from build123d import *

# Parameters (mm, degrees)
SKETCH_1_R          = 12.5
EXTRUDE_1_DEPTH     = 4
SKETCH_2_R          = 12.5
SKETCH_2_R_2        = 10
EXTRUDE_2_DEPTH     = 2.5
SKETCH_3_R          = 1.5
CUT_EXTRUDE_1_DEPTH = 52.947088465
EXTRUDE_3_DEPTH     = 25
SKETCH_5_W          = 7
SKETCH_5_H          = 5
CUT_EXTRUDE_2_DEPTH = 57.621550668
SKETCH_6_W          = 7
SKETCH_6_H          = 5
CUT_EXTRUDE_3_DEPTH = 52.780787943
EXTRUDE_6_DEPTH     = 2


with BuildPart() as part:
    # 草图1 → 凸台-拉伸1 (new body)
    with BuildSketch(Plane(origin=(0, 0, 0), x_dir=(1, 0, 0), z_dir=(0, 1, 0))):
        Circle(SKETCH_1_R)
        with BuildLine():
            Line((50, 12.5), (0, 12.5))
            ThreePointArc((0, 12.5), (8.838834765, 8.838834765), (12.5, 0))
            ThreePointArc((12.5, 0), (8.838834765, -8.838834765), (0, -12.5))
            Line((0, -12.5), (50, -12.5))
            Line((50, -12.5), (50, 12.5))
        make_face()
    extrude(amount=EXTRUDE_1_DEPTH)

    # 草图2 → 凸台-拉伸2 (add)
    with BuildSketch(Plane(origin=(0, 4, 0), x_dir=(1, 0, 0), z_dir=(0, 1, 0))):
        with Locations(Location((0, 0, 0), (0, 0, 270))):
            Circle(SKETCH_2_R)
        with Locations(Location((0, 0, 0), (0, 0, 270))):
            Circle(SKETCH_2_R_2, mode=Mode.SUBTRACT)
    extrude(amount=EXTRUDE_2_DEPTH)

    # 草图3 → 切除-拉伸1 (cut, through all)
    with BuildSketch(Plane.XZ):
        with Locations(Location((0, 0, 0), (0, 0, 270))):
            Circle(SKETCH_3_R)
        with Locations(Location((0, 7, 0), (0, 0, 270))):
            Circle(SKETCH_3_R)
        with Locations(Location((7, 0, 0), (0, 0, 270))):
            Circle(SKETCH_3_R)
        with Locations(Location((0, -7, 0), (0, 0, 270))):
            Circle(SKETCH_3_R)
        with Locations(Location((-7, 0, 0), (0, 0, 270))):
            Circle(SKETCH_3_R)
        with Locations(Location((40, 0, 0), (0, 0, 270))):
            Circle(SKETCH_3_R)
    extrude(amount=-CUT_EXTRUDE_1_DEPTH, mode=Mode.SUBTRACT)

    # 草图4 → 凸台-拉伸3 (add)
    with BuildSketch(Plane.XY.offset(12.5)):
        Polygon((50, 4), (47, 9), (33, 9), (30, 4), align=None)
    extrude(amount=-EXTRUDE_3_DEPTH)

    # 草图5 → 切除-拉伸2 (cut, through all)
    with BuildSketch(Plane.XY.offset(12.5)):
        with Locations((40, 6.5)):
            Rectangle(SKETCH_5_W, SKETCH_5_H)
    extrude(amount=-CUT_EXTRUDE_2_DEPTH, mode=Mode.SUBTRACT)

    # 草图6 → 切除-拉伸3 (cut, through all)
    with BuildSketch(Plane(origin=(0, 4, 0), x_dir=(1, 0, 0), z_dir=(0, 1, 0))):
        with Locations((40, -10)):
            Rectangle(SKETCH_6_W, SKETCH_6_H)
        with Locations((40, 10)):
            Rectangle(SKETCH_6_W, SKETCH_6_H)
    extrude(amount=-CUT_EXTRUDE_3_DEPTH, mode=Mode.SUBTRACT)

    # 草图7 → 凸台-拉伸6 (add, symmetric)
    with BuildSketch(Plane.XY):
        Polygon((30, 4), (33, 9), (12.5, 6.5), (10.351420614, 6.5), (10.351420614, 4), align=None)
    extrude(amount=EXTRUDE_6_DEPTH, both=True)


solid = part.part
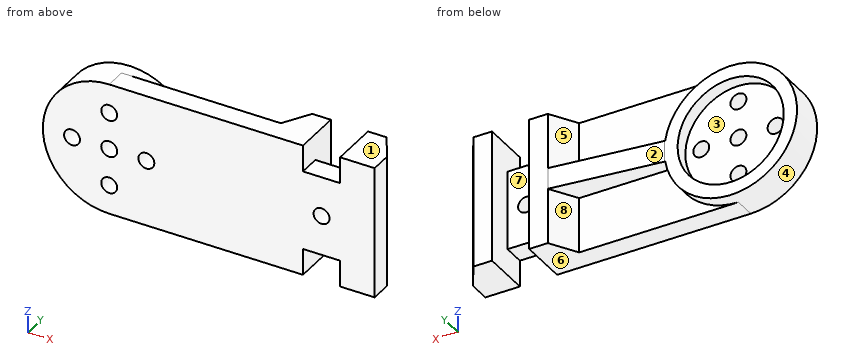
Verification items for the finished model (mm, model axes). Face numbers are marked on the shaded views. A direction names the side the tool comes from. Round coordinates to 2 decimals unless told otherwise and drop trailing zeros. Order: outer loops, then holes, each group sorted by start corner. A loop starts at its lowest first (then second) coordinate and runs counter-clockwise, first axis right, second up.
1. Section check D-D on z = -6.5. Record the cut outline in (x, y).
Final values:
outline: (-10.68, 0) - (-1.41, 0) - (-1.41, 4) - (-7.6, 4) - (-7.6, 6.5) - (-10.68, 6.5) - close; (1.41, 0) - (50, 0) - (50, 4) - (47, 9) - (43.5, 9) - (43.5, 4) - (36.5, 4) - (36.5, 9) - (33, 9) - (30, 4) - (10.68, 4) - (10.68, 6.5) - (7.6, 6.5) - (7.6, 4) - (1.41, 4) - close
2. Release check for a two-part mould opening along X. For the marked faces 1, 2 and 3 record: +X half, -X half, draft (parallel to the pull), parting line (faces both ways), or undercut.
Final values:
face 1: draft
face 2: -X half
face 3: undercut
3. Go/stop test with flat-tipped pins: P1, Ø4, axis at x = 26.5, y = 7, coming from the -Z side; P2, Ø1.5, axis at x = 26.5, y = 6, coming from the +Z side; P3, Ø2, axis at y = 6, z = 8, coming from the +X side. Record where each tip stops, or that it passes through.
Final values:
P1: stops at z = -2
P2: stops at z = 2
P3: stops at x = 49.4
4. Section check B-B on z = 0. State how many separate pieces and enclosed holes the cut face has, then the cut area to 3 significant figures.
Final values:
separate pieces: 5
enclosed holes: 0
area: 334 mm2
5. Thickness scan on L1, parallel to X at y = 2.45, z = 0; L2, parallel to Y at x = 24, z = -6.5; L3, parallel to X at y = 2.25, z = -7. Record the ranges inside material, lowest first.
Final values:
L1: x = -12.5 to -8.5, -5.5 to -1.5, 1.5 to 5.5, 8.5 to 38.5, 41.5 to 50
L2: y = 0 to 4
L3: x = -10.36 to -1.5, 1.5 to 50
6. Section check C-C on x = 40. Record the cut outline in (y, z), then the cut area to 3 significant figures.
Final values:
outline: (0, -7.5) - (4, -7.5) - (4, -1.5) - (0, -1.5) - close; (0, 1.5) - (4, 1.5) - (4, 7.5) - (0, 7.5) - close
area: 48.0 mm2
7. Section check A-A on y = 5. Record the cut outline in (x, z).
Final values:
outline: (12.34, -2) - (30.6, -2) - (30.6, -12.5) - (36.5, -12.5) - (36.5, 12.5) - (30.6, 12.5) - (30.6, 2) - (12.34, 2) arc R12.5 ccw (long way) to start; (43.5, -12.5) - (49.4, -12.5) - (49.4, 12.5) - (43.5, 12.5) - close; hole circle Ø20 at (0, 0)
8. Access from +Z, -Z, +X, -X, +Y, -Y to the whole of each face (thin tool, end or side, straight path). Record for the marked faces 4, 5, 6, 7 and 8.
Final values:
face 4: +Y
face 5: +Z, +Y
face 6: -Z, +X, -X, +Y, -Y
face 7: +Z, -Z, +Y
face 8: -Z, +Y
